```python
from build123d import *

# Parameters (mm, degrees)
SKETCH1_R           = 1.352550752
SKETCH1_RX          = 1.35255
SKETCH1_RY          = 1.352549248
BOSS_EXTRUDE2_DEPTH = 3.175


with BuildPart() as part:
    # Sketch1 → Boss-Extrude2 (new body)
    with BuildSketch(Plane.XY):
        with BuildLine():
            Line((38.098244435, 82.55), (38.098416123, -82.55))
            Line((38.098416123, -82.55), (-38.098244435, -82.55))
            Line((-38.098244435, -82.55), (-38.098244435, -31.651036949))
            add(Edge.make_bspline(
                [(-31.748247963, -25.301036949), (-38.098244435, -25.301036949), (-38.098244435, -31.651036949)],
                knots=[3.141592654, 3.141592654, 3.141592654, 4.71238898, 4.71238898, 4.71238898], degree=2, weights=[1, 0.707106781, 1]))
            Line((-31.748247963, -25.301036949), (-22.223253256, -25.301036949))
            add(Edge.make_bspline(
                [(-22.223253256, -25.301036949), (-19.04825502, -25.301036949), (-19.04825502, -22.126036949)],
                knots=[3.141592654, 3.141592654, 3.141592654, 4.71238898, 4.71238898, 4.71238898], degree=2, weights=[1, 0.707106781, 1]))
            Line((-19.04825502, -22.126036949), (-19.04825502, 22.323963051))
            add(Edge.make_bspline(
                [(-19.04825502, 22.323963051), (-19.04825502, 25.498963051), (-22.223253256, 25.498963051)],
                knots=[4.71238898, 4.71238898, 4.71238898, 6.283185307, 6.283185307, 6.283185307], degree=2, weights=[1, 0.707106781, 1]))
            Line((-22.223253256, 25.498963051), (-31.748247963, 25.498963051))
            add(Edge.make_bspline(
                [(-38.098244435, 31.848963051), (-38.098244435, 25.498963051), (-31.748247963, 25.498963051)],
                knots=[4.71238898, 4.71238898, 4.71238898, 6.283185307, 6.283185307, 6.283185307], degree=2, weights=[1, 0.707106781, 1]))
            Line((-38.098244435, 31.848963051), (-38.098244435, 82.55))
            Line((-38.098244435, 82.55), (38.098244435, 82.55))
        make_face()
        with Locations((2.505261643, -77.7875)):
            Circle(SKETCH1_R, mode=Mode.SUBTRACT)
        with Locations((-15.274748237, -77.7875)):
            Circle(SKETCH1_R, mode=Mode.SUBTRACT)
        with Locations((-33.054758116, -77.7875)):
            Circle(SKETCH1_R, mode=Mode.SUBTRACT)
        with Locations((2.505089955, 77.7875)):
            Circle(SKETCH1_R, mode=Mode.SUBTRACT)
        with Locations((-15.274919924, 77.7875)):
            Circle(SKETCH1_R, mode=Mode.SUBTRACT)
        with Locations(Location((20.298314341, -77.7875), (0, 0, -90))):
            Ellipse(SKETCH1_RX, SKETCH1_RY, mode=Mode.SUBTRACT)
        with Locations(Location((20.298142653, 77.7875), (0, 0, -90))):
            Ellipse(SKETCH1_RX, SKETCH1_RY, mode=Mode.SUBTRACT)
        with Locations(Location((-33.041827709, 77.7875), (0, 0, -90))):
            Ellipse(SKETCH1_RX, SKETCH1_RY, mode=Mode.SUBTRACT)
    extrude(amount=BOSS_EXTRUDE2_DEPTH)


solid = part.part
```
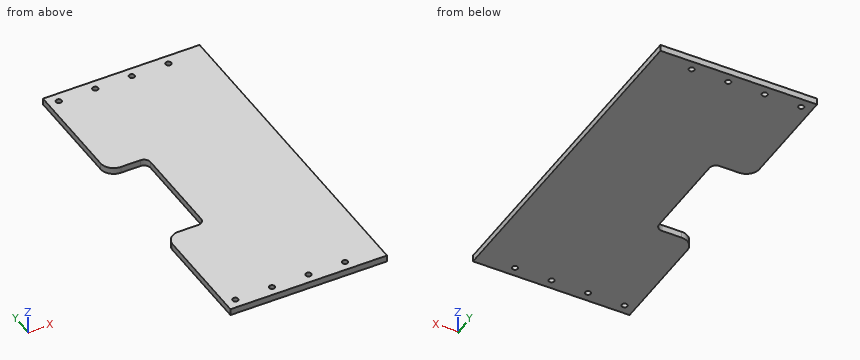
The listing builds one solid part. Answer for the finished solid, in the listing's coordinates (mm). Coordinates: 2 decimals unless noted, no trailing zeros. Order: outer loops, then holes, each group sorted by start corner. A loop starts at its lowest first (then second) coordinate and runs counter-clockwise, first axis right, second up. Notation, with made-up numbers: M -39.75,-33.75 L -0.75,-33.75 A30 cw -0.75,2.25 Z; hole C 40,-12 d11. An arc over 180 degrees is marked long. Answer as a JSON object with one key per item and string values. Group by question number.
1. Section C-C on y = 11.5 is taken. Write down the section's boundary in (x, z) (3 decimals).
2. Section A-A on x = -25.5 is taken. Write down the section's boundary in (y, z) (3 decimals), then the cut area to 3 significant figures.
3. Straight lines are drawn through the part: line 1 (Y direction, x = -30, z = 2.3); line 2 (X direction, y = 31.5, z = 0.5); line 3 (X direction, y = -19, z = 1.1). For each, find the intervals that lie inside material, in ascending order.
4. A flat-ended cylindrical pin translates along its axis: P1, Ø1.6, axis at x = 2.51, y = 77.79, coming from the +Z side. Find the tip coordinate at first contact, or state that the pin passes through.
5. Section B-B on z = 1.4 is taken. State how many separate pieces and enclosed holes the cut face has, then the cut area to 3 significant figures.
Values follow:
{
 "1": {"outline": "M -19.048,0 L 38.098,0 L 38.098,3.175 L -19.048,3.175 Z"},
 "2": {"outline": "M -82.55,0 L -25.301,0 L -25.301,3.175 L -82.55,3.175 Z; M 25.499,0 L 82.55,0 L 82.55,3.175 L 25.499,3.175 Z", "area": "363 mm2"},
 "3": {"line 1": "-82.55 to -25.3, 25.5 to 82.55", "line 2": "-38.09 to 38.1", "line 3": "-19.05 to 38.1"},
 "4": {"P1": "through"},
 "5": {"separate pieces": "1", "enclosed holes": "8", "area": "11,600 mm2"}
}
